Here's how the part is built. I have some questions about the finished solid (model axes, mm). A direction names the side the tool comes from. Coordinates: 2 decimals unless noted, no trailing zeros. Loops run counter-clockwise (first coordinate to the right, second up) from the corner with the lowest first, then second, coordinate; pieces in that order, holes last. Notation, with made-up numbers: (-39.5, -25) -> (-15.5, -25) arc R33 cw to (-15.5, 6) -> close; hole circle Ø2 at (55, 30). An arc over 180 degrees is marked (long way). Answer as a JSON object with one key per item and string values. Group by question number.
1) I want a section at A-A (x = 39). Write out the boundary of the cut face in (y, z) (3 decimals).
2) I want a section at B-B (z = 14.5). Write out the boundary of the cut face in (x, y).
3) I'm going to push flat-ended pins straight in: pin 1 (1.5 mm diameter, centred on x = -39, y = -14.5, fed in from +Z); pin 2 (1.6 mm diameter, centred on x = -52, y = -59, fed in from -Z); pin 3 (2 mm diameter, centred on x = 51.5, y = 58.5, fed in from -Z). Where does each tip first touch, or does it pass through?
4) If we mould it in two halves opening along X, with no side actions, what happens to faces 1 (the flat face through (-80, 18, 1)), 2 (the flat face through (1, -58, 15)), 3 (the cylindrical face through (30, 59, 15))? For each: +X half, -X half, draft (parallel to the pull), parting line (faces both ways), or undercut.
5) I need wall thicknesses on probe 1 along Y at (x, z) = (-68.5, 5.75); probe 2 along Z at (x, y) = (18.5, -38); probe 3 along Y at (x, z) = (-63, 3.25). Which ranges of each line are inside material? Lowest first, please. Write a range as [from, to].
6) I want a section at D-D (y = 20). Write out the boundary of the cut face in (x, z).
7) Which directions (+Z, -Z, +X, -X, +Y, -Y) give clear straight access to the entire face, cutting with the end or side of a thin tool? Please do faces 4 (the flat face through (-1, 60, 15)), 5 (the cylindrical face through (70, 59, 15)), 6 (the flat face through (-1, 1, 2)).
8) I want a section at C-C (x = 16). Write out the boundary of the cut face in (y, z), then the cut area to 3 significant figures.
Autodesk Inventor part; units mm, degrees
ref_plane "YZ Plane" through (0, 0, 0) normal (1, 0, 0) x (0, 1, 0)
ref_plane "XZ Plane" through (0, 0, 0) normal (0, 1, 0) x (-1, 0, 0)
ref_plane "XY Plane" through (0, 0, 0) normal (0, 0, 1) x (1, 0, 0)
sketch "Sketch1" plane through (0, 0, 0) normal (0, 0, 1) x (1, 0, 0)
  line L0 (-80, -60) -> (80, -60)
  line L1 (80, -60) -> (80, 60)
  line L2 (80, 60) -> (-80, 60)
  line L3 (-80, 60) -> (-80, -60)
  line L4 (-80, -60) -> (80, 60) construction
  line L5 (80, -60) -> (-80, 60) construction
  point P0 (0, 0)
  dimension "d0" = 160
  dimension "d1" = 120
extrude "Plate1" add sketch "Sketch1" along normal blind 2
sketch "Sketch2" plane through (0, 0, 0) normal (0, 0, -1) x (-1, 0, 0)
  line L0 (-60, 40) -> (140, 40) construction
  line L1 (140, 40) -> (140, 20) construction
  line L2 (140, 20) -> (-60, 20) construction
  line L3 (-60, 20) -> (-60, 40) construction
  line L4 (-80, 60) -> (80, 60)
  line L5 (-80, -60) -> (-80, 60)
  point P0 (0, 0)
  point P1 (-48, 100)
  point P2 (-50, 98)
  dimension "d6" = 200
  dimension "d9" = 20
  dimension "d10" = 20
  dimension "d11" = 20
mark "Mark1"
sketch "Sketch3" plane through (80, 58, 0) normal (0, 1, 0) x (-1, 0, 0)
  line L0 (160, 0) -> (0, 0)
  line L1 (0, 0) -> (0, -25)
  line L2 (0, -25) -> (160, -25)
  line L3 (160, -25) -> (160, 0)
edge flange "Flange1" height 25 angle 90 thickness 2 bend radius 2.75 thickness toward (0, 1, 0) relief round relief width 2 relief depth 1 corner gap 2.75 corner form 0 edges at (0, 60, 0) (0, -60, 0) wall of the first edge with corners at (-80, 58, 0) (80, 58, 0) (80, 58, 25) (-80, 58, 25)
bend "Bend1"
corner "Corner1"
sketch "Sketch4" plane through (0, 0, 0) normal (0, 1, 0) x (-1, 0, 0)
  line L0 (-80, 4.75) -> (80, 4.75) construction
  line L1 (80, 4.75) -> (80, 25)
  line L2 (80, 25) -> (-80, 25) construction
  line L3 (-80, 4.75) -> (-80, 25)
  line L4 (-65, 14.875) -> (-35, 14.875) construction
  line L5 (-65, 9.875) -> (-35, 9.875)
  line L6 (-35, 19.875) -> (-65, 19.875)
  arc A0 (-65, 19.875) -> (-65, 9.875) centre (-65, 14.875) ccw
  arc A1 (-35, 9.875) -> (-35, 19.875) centre (-35, 14.875) ccw
  line L7 (35, 14.875) -> (65, 14.875) construction
  line L8 (35, 9.875) -> (65, 9.875)
  line L9 (65, 19.875) -> (35, 19.875)
  arc A2 (35, 19.875) -> (35, 9.875) centre (35, 14.875) ccw
  arc A3 (65, 9.875) -> (65, 19.875) centre (65, 14.875) ccw
  line L10 (0, 4.75) -> (0, 25) construction
  point P0 (0, 0)
  point P1 (-50, 14.875)
  point P2 (50, 14.875)
  point P3 (-80, 14.875)
  dimension "d22" = 30
  dimension "d23" = 10
  dimension "d24" = 100
extrude "Extrusion1" cut sketch "Sketch4" along normal through all both and the other way through all
fillet "Corner Round1" radius 6 2 edges at (80, 59, 25) (80, -59, 25)
equation "\"d2\" = Thickness"
equation "\"d12\" = BendReliefWidth"
equation "\"d13\" = BendReliefDepth"
equation "\"d14\" = MinimumRemnant"
equation "\"d15\" = TransitionRadius"
equation "\"d18\" = BendRadius"
equation "\"d19\" = CornerReliefSize"
equation "\"d20\" = GapSize"
equation "\"d21\" = JacobiRadiusSize"
equation "\"BendReliefWidth\" = Thickness"
equation "\"BendReliefDepth\" = 0.5 * Thickness"
equation "\"CornerReliefSize\" = 4 * Thickness"
equation "\"MinimumRemnant\" = 2 * Thickness"
equation "\"TransitionRadius\" = BendRadius"
equation "\"JacobiRadiusSize\" = BendRadius"
equation "\"GapSize\" = Thickness"
properties part number "TRM 026 right board damper" material "AISI 304"
Determined:
{
 "1": {"outline": "(-60, 4.75) arc R4.75 ccw to (-55.25, 0) -> (55.25, 0) arc R4.75 ccw to (60, 4.75) -> (60, 9.875) -> (58, 9.875) -> (58, 4.75) arc R2.75 cw to (55.25, 2) -> (-55.25, 2) arc R2.75 cw to (-58, 4.75) -> (-58, 9.875) -> (-60, 9.875) -> close; (-60, 19.875) -> (-58, 19.875) -> (-58, 25) -> (-60, 25) -> close; (58, 19.875) -> (60, 19.875) -> (60, 25) -> (58, 25) -> close"},
 "2": {"outline": "(-80, -60) -> (-69.99, -60) -> (-69.99, -58) -> (-80, -58) -> close; (-80, 58) -> (-69.99, 58) -> (-69.99, 60) -> (-80, 60) -> close; (-30.01, -60) -> (30.01, -60) -> (30.01, -58) -> (-30.01, -58) -> close; (-30.01, 58) -> (30.01, 58) -> (30.01, 60) -> (-30.01, 60) -> close; (69.99, -60) -> (80, -60) -> (80, -58) -> (69.99, -58) -> close; (69.99, 58) -> (80, 58) -> (80, 60) -> (69.99, 60) -> close"},
 "3": {"pin 1": "z = 2", "pin 2": "z = 1.03", "pin 3": "z = 0.57"},
 "4": {"face 1": "-X half", "face 2": "draft", "face 3": "undercut"},
 "5": {"probe 1": "[-60, -58], [58, 60]", "probe 2": "[0, 2]", "probe 3": "[-59.76, -57.55], [57.55, 59.76]"},
 "6": {"outline": "(-80, 0) -> (80, 0) -> (80, 2) -> (-80, 2) -> close"},
 "7": {"face 4": "+Z, -Z, +X, -X, +Y", "face 5": "+Y, -Y", "face 6": "+Z, +X, -X"},
 "8": {"outline": "(-60, 4.75) arc R4.75 ccw to (-55.25, 0) -> (55.25, 0) arc R4.75 ccw to (60, 4.75) -> (60, 25) -> (58, 25) -> (58, 4.75) arc R2.75 cw to (55.25, 2) -> (-55.25, 2) arc R2.75 cw to (-58, 4.75) -> (-58, 25) -> (-60, 25) -> close", "area": "326 mm^2"}
}
